Autodesk Inventor part; units mm, degrees
ref_plane "YZ Plane" through (0, 0, 0) normal (1, 0, 0) x (0, 1, 0)
ref_plane "XZ Plane" through (0, 0, 0) normal (0, 1, 0) x (-1, 0, 0)
ref_plane "XY Plane" through (0, 0, 0) normal (0, 0, 1) x (1, 0, 0)
sketch "Skizze1" plane through (0, 0, 0) normal (0, 0, 1) x (1, 0, 0)
  circle A0 centre (0, 0) radius 2
  circle A1 centre (0, 0) radius 9.6
  circle A2 centre (0, 0) radius 6.35 construction
  circle A3 centre (6.35, 0) radius 1.4
  circle A4 centre (-6.35, 0) radius 1.4
  circle A5 centre (0, 6.35) radius 1.4
  circle A6 centre (0, -6.35) radius 1.4
  circle A7 centre (0, 0) radius 11.6
  circle A8 centre (0, 0) radius 4.3516
  line L0 (0, 16.24) -> (0, -16.24) construction
  line L1 (-16.24, 0) -> (16.24, 0) construction
  dimension "d0" = 19.2
  dimension "d1" = 12.7
  dimension "d2" = 2.8
  dimension "d3" = 4
  dimension "d4" = 2
  dimension "d5" = 8.7031
extrude "Extrusion1" add sketch "Skizze1" along normal blind 2 contours A1 | A7 | A8
extrude "Extrusion2" add sketch "Skizze1" along normal blind 5 from surface at 2 contours A7
sketch "Skizze2" plane through (0, 0, 0) normal (0, 1, 0) x (-1, 0, 0)
  circle A0 centre (0, 4.5) radius 1.25
  line L0 (9.6, 7) -> (-9.6, 7)
  point P0 (0, 0)
  dimension "d10" = 2.5
  dimension "d11" = 2.5
extrude "Extrusion3" cut sketch "Skizze2" against normal through all
properties part number "Input"
The listing builds one solid part. Answer for the finished solid, in the listing's coordinates (mm). A direction names the side the tool comes from. Give positions to 0.01 mm unless a question says otherwise; leave off trailing zeros. Order: outer loops, then holes, each group sorted by start corner. A loop starts at its lowest first (then second) coordinate and runs counter-clockwise, first axis right, second up. Notation, with made-up numbers: (-20.75, 78) -> (3.25, 78) arc R24 ccw to (3.25, 101) -> close; hole circle Ø5 at (88, -38). An arc over 180 degrees is marked (long way). Answer as a JSON object with one key per item and string values. Group by question number.
Item 1: Determine the mould class of faces 1 (the cylindrical face through (0, 2, 1)), 2 (the cylindrical face through (-11.59, -0.51, 3.45)), 3 (the flat face through (2.4, 0.2, 0)) for opening direction X: pulls with the +X half, pulls with the -X half, needs draft (parallel to the pull), parting line crosses it, or undercut.
Item 2: A flat-ended cylindrical pin translates along its axis: pin 1 (4 mm diameter, centred on y = -6.5, z = 4.5, fed in from +X). Find the tip coordinate at first contact, or state that the pin passes through.
Item 3: The part is cut by section A-A on x = 0. Write down the section's boundary in (y, z), and give its area (3 significant figures).
Item 4: Consider L1, parallel to Y at x = 0, z = 0.4; L2, parallel to Y at x = -1.75, z = 2.25; L3, parallel to X at y = -1.5, z = 1.75. Determine where each line is inside the solid, lowest interval first. Write a range as from..to.
Item 5: The part is cut by section D-D on y = -0.5. Write down the section's boundary in (x, z), and give its area (3 significant figures).
Item 6: A tool of negligible diameter and unlimited length cuts with its end or side. For faces 4 (the cylindrical face through (-0.18, -7.74, 0.99)), 5 (the cylindrical face through (5.161, -8.095, 4.465)), 6 (the cylindrical face through (0.27, -10.54, 3.28)), from which of +Z, -Z, +X, -X, +Y, -Y can it reach the whole face along a straight path? Write none if from no direction.
Item 7: The part is cut by section B-B on z = 0.75. Write down the section's boundary in (x, y), and give its area (3 significant figures).
Item 8: The part is cut by section C-C on y = 6.35. Write down the section's boundary in (x, z).
Result set:
{
 "1": {"face 1": "undercut", "face 2": "parting line crosses it", "face 3": "needs draft"},
 "2": {"pin 1": "x = 10.69"},
 "3": {"outline": "(-11.6, 0) -> (-7.75, 0) -> (-7.75, 2) -> (-9.6, 2) -> (-9.6, 3.25) -> (-11.6, 3.25) -> close; (-11.6, 5.75) -> (-9.6, 5.75) -> (-9.6, 7) -> (-11.6, 7) -> close; (-4.95, 0) -> (-2, 0) -> (-2, 2) -> (-4.95, 2) -> close; (2, 0) -> (4.95, 0) -> (4.95, 2) -> (2, 2) -> close; (7.75, 0) -> (11.6, 0) -> (11.6, 7) -> (9.6, 7) -> (9.6, 2) -> (7.75, 2) -> close", "area": "42.2 mm²"},
 "4": {"L1": "-11.6..-7.75, -4.95..-2, 2..4.95, 7.75..11.6", "L2": "-11.47..-9.44, 9.44..11.47", "L3": "-11.5..-1.32, 1.32..11.5"},
 "5": {"outline": "(-11.59, 0) -> (-7.66, 0) -> (-7.66, 2) -> (-9.59, 2) -> (-9.59, 7) -> (-11.59, 7) -> close; (-5.04, 0) -> (-1.94, 0) -> (-1.94, 2) -> (-5.04, 2) -> close; (1.94, 0) -> (5.04, 0) -> (5.04, 2) -> (1.94, 2) -> close; (7.66, 0) -> (11.59, 0) -> (11.59, 7) -> (9.59, 7) -> (9.59, 2) -> (7.66, 2) -> close", "area": "48.2 mm²"},
 "6": {"face 4": "+Z, -Z", "face 5": "+Z", "face 6": "-Y"},
 "7": {"outline": "circle Ø23.2 at (0, 0); hole circle Ø2.8 at (-6.35, 0); hole circle Ø4 at (0, 0); hole circle Ø2.8 at (0, -6.35); hole circle Ø2.8 at (0, 6.35); hole circle Ø2.8 at (6.35, 0)", "area": "386 mm²"},
 "8": {"outline": "(-9.71, 0) -> (-1.4, 0) -> (-1.4, 2) -> (-7.2, 2) -> (-7.2, 7) -> (-9.71, 7) -> close; (1.4, 0) -> (9.71, 0) -> (9.71, 7) -> (7.2, 7) -> (7.2, 2) -> (1.4, 2) -> close"}
}
